Read the model definition and answer for the solid it produces. Units are mm, in the model's axes. Face numbers are marked on the shaded views. A direction names the side the tool comes from. Coordinates: 2 decimals unless noted, no trailing zeros. Write each loop counter-clockwise with the first axis right and the second up, starting at its lowest first coordinate (ties: lowest second). Pieces come first, ordered by that corner, then holes. Notation, with made-up numbers: (-28.75, 5) -> (-24.75, 5) arc R25 cw to (-24.75, 44) -> close; hole circle Ø10 at (20, 21.5). An arc over 180 degrees is marked (long way). Write item = value, one per line. Start each with the question number.
1) Flat-ended cylindrical pins translate along their axes: pin 1 Ø5 at (y, z) = (-57.5, 11) entering from +X; pin 2 Ø1.5 at (y, z) = (-59, -37) entering from -X; pin 3 Ø2 at (x, z) = (-10.5, 13) entering from -Y. Find the tip coordinate at first contact, or state that the pin passes through.
2) Find the intervals of material crossed by line 1 along X through (y, z) = (-36, -16); line 2 along Z through (x, y) = (6, -25); line 3 along X through (y, z) = (-76, -13), in increasing order. Write a range as from..to.
3) Section C-C (x = 7) is taken. Determine the outline of the cut face in (y, z).
4) Section A-A (y = -9.5) is taken. Determine the outline of the cut face in (x, z), plus the area to 3 significant figures.
5) A tool of negligible diameter and unlimited length cuts with its end or side. For the marked faces 1 and 2, from which of +Z, -Z, +X, -X, +Y, -Y can it reach the whole face along a straight path? Write none if from no direction.
6) Section B-B (z = -12) is taken. Determine the outline of the cut face in (x, y), plus the area to 4 significant figures.
7) For a pull along X with two mould halves and no side action, classify the marked faces 3, 4, 5 and 6 as released by +X, released by -X, zero draft, split by the parting line, or undercut.
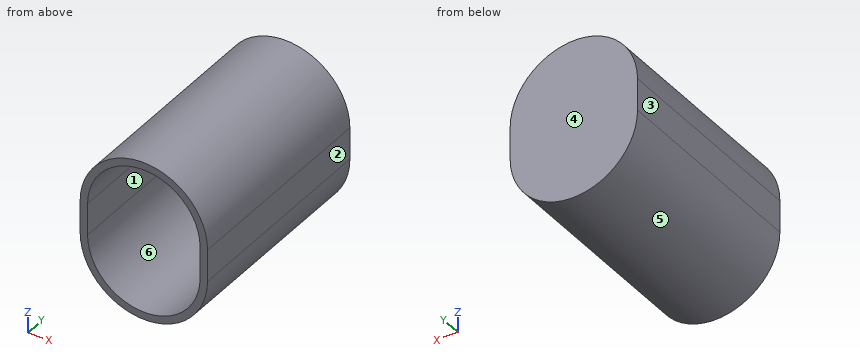
from build123d import *

# Parameters (mm, degrees)
F1_DEPTH = 100
F2_T     = -3.5


with BuildPart() as f1:
    # F0 (on Front) → F1 (new body)
    with BuildSketch(Plane.XZ):
        with BuildLine():
            Line((35.748127, -15), (35.748127, 0))
            ThreePointArc((35.748127, 0), (5.748127, 30), (-24.251873, 0))
            Line((-24.251873, 0), (-24.251873, -15))
            ThreePointArc((-24.251873, -15), (5.748127, -45), (35.748127, -15))
        make_face()
    extrude(amount=F1_DEPTH)

    # F2
    f2_openings = [f1.faces().sort_by_distance(p)[0] for p in [
        (5.748127, -100, -7.5),
    ]]
    offset(amount=F2_T, openings=f2_openings)


solid = f1.part
Answer key:
q1.pin_1 = 34.52
q1.pin_2 = -15.43
q1.pin_3 = -3.5
q2.line_1 = -24.24..-20.73, 32.23..35.73
q2.line_2 = -45..-41.5, 26.5..30
q2.line_3 = -24.25..-20.75, 32.25..35.75
q3.outline = (-100, -44.97) -> (0, -44.97) -> (0, 29.97) -> (-100, 29.97) -> (-100, 26.47) -> (-3.5, 26.47) -> (-3.5, -41.47) -> (-100, -41.47) -> close
q4.outline = (-24.25, -15) arc R30 ccw to (35.75, -15) -> (35.75, 0) arc R30 ccw to (-24.25, 0) -> close; hole (-20.75, -15) arc R26.5 ccw to (32.25, -15) -> (32.25, 0) arc R26.5 ccw to (-20.75, 0) -> close
q4.area = 726 mm^2
q5.face_1 = -Y
q5.face_2 = +Z, -Z, +X, +Y, -Y
q6.outline = (-24.25, -100) -> (-20.75, -100) -> (-20.75, -3.5) -> (32.25, -3.5) -> (32.25, -100) -> (35.75, -100) -> (35.75, 0) -> (-24.25, 0) -> close
q6.area = 885.5 mm^2
q7.face_3 = released by -X
q7.face_4 = zero draft
q7.face_5 = split by the parting line
q7.face_6 = undercut
